Input: part model. Units: mm. Frame: model coordinates. Coordinates: 2 decimals unless noted, no trailing zeros. Loops run counter-clockwise (first coordinate to the right, second up) from the corner with the lowest first, then second, coordinate; pieces in that order, holes last. Notation, with made-up numbers: M -36,9.5 L 19,9.5 A31 cw 19,45.5 Z; hole C 36.25,69.25 d5. An arc over 180 degrees is marked long. Use a Markdown table: item, result. Add a question column.
1. Pin query (flat end, axial travel): pin 1 (1.5 mm diameter, centred on y = 28, z = 1.5, fed in from +X); pin 2 (3 mm diameter, centred on x = -55.5, z = 3.5, fed in from +Y) (3 decimals); pin 3 (3 mm diameter, centred on x = 20, z = 4, fed in from +Y). Return the tip coordinate at first contact, or that it passes through.
2. Section C-C on y = 38.5. Output: boundary loops of the cut face in (x, z).
3. Line query: L1, parallel to X at y = 1.5, z = 1.5; L2, parallel to Y at x = 1, z = 2.5 (1 decimal); L3, parallel to Y at x = 0, z = 2 (1 decimal). Output: solid intervals per line, ascending. Write a range as [from, to].
4. Section A-A on z = 2.25. State how many separate pieces and enclosed holes the cut face has, then the cut area to 3 significant figures.
5. Section D-D on y = 0. Output: boundary loops of the cut face in (x, z), then the cut area to 3 significant figures.
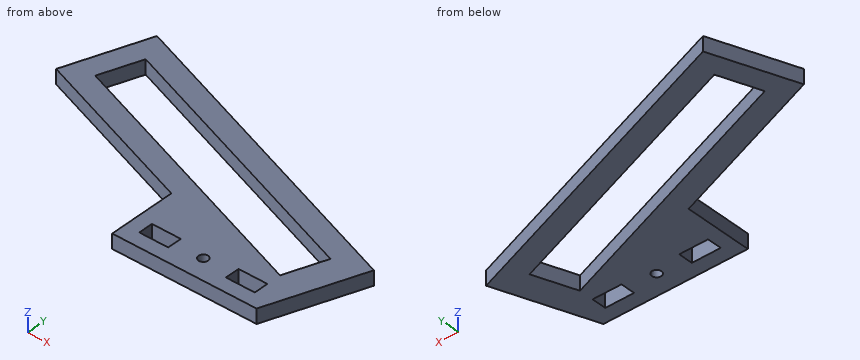
```python
from build123d import *

# Parameters (mm, degrees)
SKETCH1_W               = 63.5
SKETCH1_H               = 19.05
BOSS_EXTRUDE1_DEPTH     = 6.35
SKETCH2_R               = 2.0955
SKETCH2_W               = 12.7
SKETCH2_H               = 6.35
CUT_EXTRUDE1_DEPTH      = 6.35
BOSS_EXTRUDE2_START     = -6.35
BOSS_EXTRUDE2_OUTLINE_W = 12.7
BOSS_EXTRUDE2_OUTLINE_H = 6.35
BOSS_EXTRUDE2_OUTLINE_R = 2.0955
BOSS_EXTRUDE2_DEPTH     = 6.35


with BuildPart() as part:
    # Sketch1 → Boss-Extrude1 (new body)
    with BuildSketch(Plane.XY):
        Rectangle(SKETCH1_W, SKETCH1_H)
    extrude(amount=BOSS_EXTRUDE1_DEPTH)

    # Sketch2 → Cut-Extrude1 (cut)
    with BuildSketch(Plane.XY.offset(6.35)):
        Circle(SKETCH2_R)
        with Locations((-19.05, 0)):
            Rectangle(SKETCH2_W, SKETCH2_H)
        with Locations((19.05, 0)):
            Rectangle(SKETCH2_W, SKETCH2_H)
    extrude(amount=-CUT_EXTRUDE1_DEPTH, mode=Mode.SUBTRACT)

    # Boss-Extrude2: read off the stored shape, not the designer's step
    # Boss-Extrude2 outline → Boss-Extrude2 (add)
    with BuildSketch(Plane.XY.offset(6.35).offset(BOSS_EXTRUDE2_START)):
        Polygon((-31.75, 20.189605605), (-31.75, -9.525), (31.75, -9.525), (46.902968685, 32.107439299), (-93.118309457, 83.071016706), (-106.149276918, 47.268727855), align=None)
        with Locations((-19.05, 0)):
            Rectangle(BOSS_EXTRUDE2_OUTLINE_W, BOSS_EXTRUDE2_OUTLINE_H, mode=Mode.SUBTRACT)
        Circle(BOSS_EXTRUDE2_OUTLINE_R, mode=Mode.SUBTRACT)
        with Locations((19.05, 0)):
            Rectangle(BOSS_EXTRUDE2_OUTLINE_W, BOSS_EXTRUDE2_OUTLINE_H, mode=Mode.SUBTRACT)
        Polygon((-87.425479109, 70.862702628), (31.91548373, 27.426144426), (25.4, 9.525), (-93.94096284, 52.961558202), align=None, mode=Mode.SUBTRACT)
    extrude(amount=BOSS_EXTRUDE2_DEPTH)


solid = part.part
```
Answers below:
| question | item | result |
|---|---|---|
| 1 | pin 1 | stops at x = 45.68 |
| 1 | pin 2 | stops at y = 69.925 |
| 1 | pin 3 | stops at y = 42.45 |
| 2 | outline | M -82.06,0 L -54.21,0 L -54.21,6.35 L -82.06,6.35 Z; M 1.49,0 L 29.34,0 L 29.34,6.35 L 1.49,6.35 Z |
| 3 | L1 | x = [-31.75, -25.4], [-12.7, -1.46], [1.46, 12.7], [25.4, 35.76] |
| 3 | L2 | y = [-9.5, -1.8], [1.8, 18.4], [38.7, 48.8] |
| 3 | L3 | y = [-9.5, -2.1], [2.1, 18.8], [39, 49.2] |
| 4 | separate pieces | 1 |
| 4 | enclosed holes | 4 |
| 4 | area | 4,240 mm² |
| 5 | outline | M -31.75,0 L -25.4,0 L -25.4,6.35 L -31.75,6.35 Z; M -12.7,0 L -2.1,0 L -2.1,6.35 L -12.7,6.35 Z; M 2.1,0 L 12.7,0 L 12.7,6.35 L 2.1,6.35 Z; M 25.4,0 L 35.22,0 L 35.22,6.35 L 25.4,6.35 Z |
| 5 | area | 237 mm² |
